Part print with two shaded views. Sizes in mm from the minimum x, y, z corner. Give positions to 0.01 mm unless a question says otherwise; leave off trailing zeros. Order: outer loops, then holes, each group sorted by start corner. A loop starts at its lowest first (then second) coordinate and runs counter-clockwise, first axis right, second up. Notation, with made-up numbers: M -16.5,24 L -6.5,24 A23 ccw -6.5,60 Z; hole C -3.5,-12 d6. An arc over 180 degrees is marked long. Return JSON: item names as keys, results as strings.
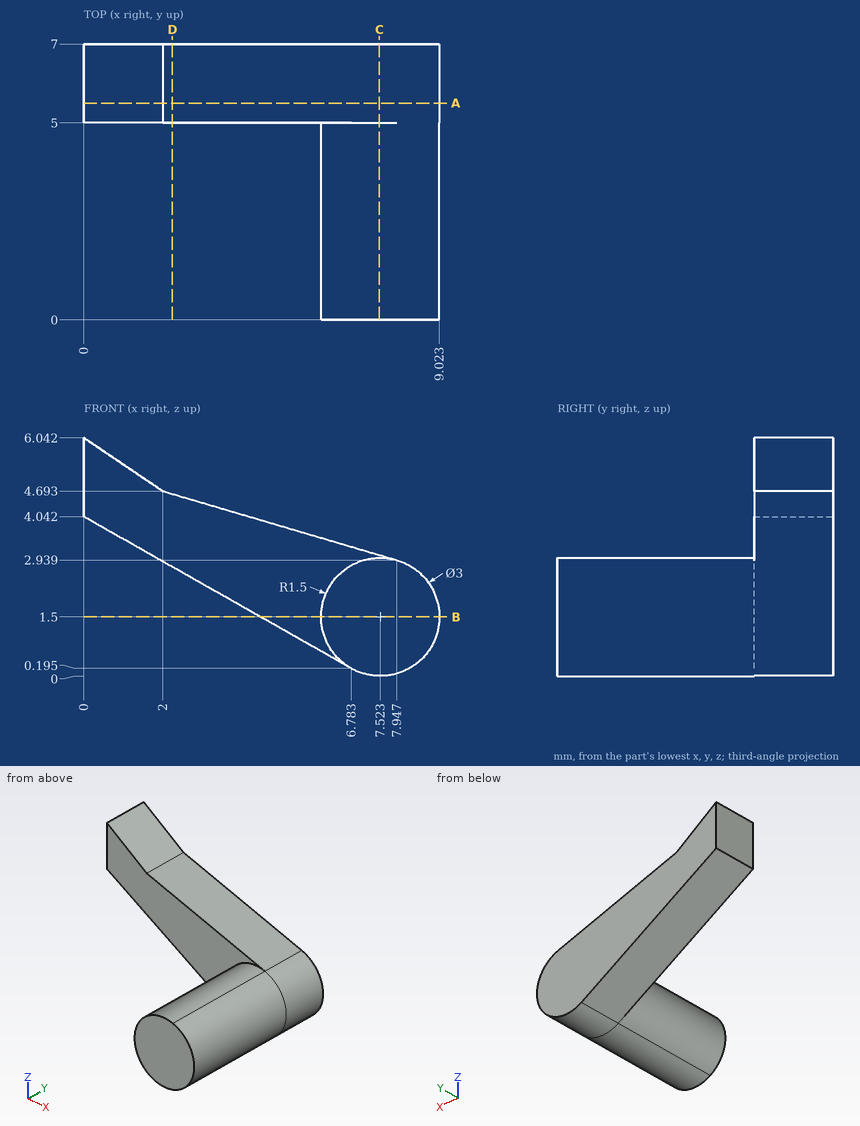
Q1. Band-saw the part on B-B (z = 1.5). Give the cut face in (x, y), then the cut area to 3 significant figures.
Established:
{"outline": "M 4.48,5 L 6.02,5 L 6.02,0 L 9.02,0 L 9.02,7 L 4.48,7 Z", "area": "24.1 mm²"}
Q2. Pin check, flat tips, straight feed: pin 1 (1 mm diameter, centred on x = 6.5, z = 3.5, fed in from -Y); pin 2 (1.5 mm diameter, centred on y = 3, z = 3.5, fed in from +X); pin 3 (1.5 mm diameter, centred on y = 3, z = 2.5, fed in from -X). Stop position of each tip, or through.
Established:
{"pin 1": "stops at y = 5", "pin 2": "stops at x = 8.35", "pin 3": "stops at x = 6.04"}
Q3. Band-saw the part on A-A (y = 5.5). Give the cut face in (x, z) (1 decimal).
Established:
{"outline": "M 0,4 L 6.8,0.2 A1.5 ccw long 7.9,2.9 L 2,4.7 L 0,6 Z"}
Q4. Probe line 1 along Y through (x, z) = (5, 2.5); line 2 along Z through (x, y) = (0.5, 6.5) (1 decimal); line 3 along Z through (x, y) = (6.5, 2.5) (1 decimal). List the from-to ranges inside material, lowest first.
Established:
{"line 1": "y = 5 to 7", "line 2": "z = 3.8 to 5.7", "line 3": "z = 0.4 to 2.6"}
Q5. Band-saw the part on C-C (x = 7.5). Give the cut face in (y, z).
Established:
{"outline": "M 0,0 L 7,0 L 7,3.07 L 5,3.07 L 5,3 L 0,3 Z"}
Q6. Band-saw the part on D-D (x = 2.25). Give the cut face in (y, z).
Established:
{"outline": "M 5,2.77 L 7,2.77 L 7,4.62 L 5,4.62 Z"}
